Can you work these out from the model? Positions are in its coordinate system, mm. A direction names the side the tool comes from. Give positions to 0.01 mm unless a question says otherwise; leave off trailing zeros. Order: outer loops, then holes, each group sorted by start corner. A loop starts at its lowest first (then second) coordinate and runs counter-clockwise, first axis right, second up. Notation, with made-up numbers: (-18.75, 33.5) - (-5.75, 33.5) arc R16 ccw to (-5.75, 56.5) - close; hole circle Ø7 at (-10, 3.25). An arc over 180 degrees is marked (long way). One line per question, with ' | ' between items.
```python
from build123d import *

# Parameters (mm, degrees)
PAD012_DEPTH            = 3
FILLET037_R             = 3.35
SKETCH185_R             = 1.15
POCKET053_DEPTH         = 3
POCKET056_DEPTH         = 5
SKETCH189_W             = 32
SKETCH189_H             = 20
POCKET057_DEPTH         = 1.5
BODY024_PLACEMENT_ANGLE = 149


with BuildPart() as part:
    # Sketch184 → Pad012 (new body)
    with BuildSketch(Plane(origin=(0, 0, 0), x_dir=(1, 0, 0), z_dir=(0, 0, -1))):
        Polygon((101.467362, -402.500006), (130.400002, -402.500006), (135.400002, -402.500006), (135.400002, -397.500006), (174.999975, -357.90402), (174.999975, -245), (289.999995, -245), (294.999995, -245), (294.999995, -215), (289.999995, -215), (224.999995, -215), (224.999995, -199.999997), (219.999995, -199.999997), (199.999995, -199.999997), (194.999995, -199.999997), (194.999995, -215.000003), (168.459985, -215.000003), (161.999993, -198.359996), (161.999993, -115.000006), (161.999993, -110.000006), (156.999993, -110.000006), (134.576923, -122.534363), (131.999997, -126.895911), (131.999997, -200.027011), (144.989344, -239.967928), (144.989344, -343.839368), (96.467362, -392.500006), (96.467362, -397.500006), (96.467362, -402.500006), align=None)
    extrude(amount=PAD012_DEPTH)

    # Fillet037
    fillet037_edges = [part.edges().sort_by_distance(p)[0] for p in [
        (194.999995, 215.000003, -1.5),
        (168.459985, 215.000003, -1.5),
        (161.999993, 198.359996, -1.5),
        (161.999993, 110.000006, -1.5),
        (156.999993, 110.000006, -1.5),
        (134.576923, 122.534363, -1.5),
        (131.999997, 126.895911, -1.5),
        (131.999997, 200.027011, -1.5),
        (144.989344, 239.967928, -1.5),
        (144.989344, 343.839368, -1.5),
        (96.467362, 392.500006, -1.5),
        (135.400002, 397.500006, -1.5),
        (174.999975, 357.90402, -1.5),
        (174.999975, 245, -1.5),
        (294.999995, 245, -1.5),
        (294.999995, 215, -1.5),
        (224.999995, 215, -1.5),
    ]]
    fillet(fillet037_edges, radius=FILLET037_R)

    # Sketch185 (on Face5 of Fillet037) → Pocket053 (cut)
    with BuildSketch(Plane(origin=(0, 0, -3), x_dir=(1, 0, 0), z_dir=(0, 0, -1))):
        with Locations((105, -389)):
            Circle(SKETCH185_R)
        with Locations((145, -349)):
            Circle(SKETCH185_R)
        with Locations((147.500002, -309.000005)):
            Circle(SKETCH185_R)
        with Locations((147.500002, -259.000004)):
            Circle(SKETCH185_R)
        with Locations((172.500003, -259.000004)):
            Circle(SKETCH185_R)
        with Locations((172.500003, -309.000005)):
            Circle(SKETCH185_R)
        with Locations((172.500003, -349.000005)):
            Circle(SKETCH185_R)
        with Locations((147.665007, -382.765018)):
            Circle(SKETCH185_R)
        with Locations((178.000003, -242.500004)):
            Circle(SKETCH185_R)
        with Locations((218.000003, -242.500004)):
            Circle(SKETCH185_R)
        with Locations((258.000004, -242.500004)):
            Circle(SKETCH185_R)
        with Locations((258.000004, -217.500003)):
            Circle(SKETCH185_R)
        with Locations((292, -242.500004)):
            Circle(SKETCH185_R)
        with Locations((292.000004, -217.500003)):
            Circle(SKETCH185_R)
        with Locations((292.500004, -230.000003)):
            Circle(SKETCH185_R)
        with Locations((223.000003, -217.000003)):
            Circle(SKETCH185_R)
        with Locations((197, -217)):
            Circle(SKETCH185_R)
        with Locations((166.109996, -217.109995)):
            Circle(SKETCH185_R)
        with Locations((147.500002, -239)):
            Circle(SKETCH185_R)
        with Locations((141, -220)):
            Circle(SKETCH185_R)
        with Locations((134.427551, -201)):
            Circle(SKETCH185_R)
        with Locations((160.149996, -200.999996)):
            Circle(SKETCH185_R)
        with Locations((134.427551, -161)):
            Circle(SKETCH185_R)
        with Locations((159.500002, -161.000002)):
            Circle(SKETCH185_R)
        with Locations((137, -124)):
            Circle(SKETCH185_R)
        with Locations((146.849997, -118.149997)):
            Circle(SKETCH185_R)
        with Locations((159, -113)):
            Circle(SKETCH185_R)
    extrude(amount=-POCKET053_DEPTH, mode=Mode.SUBTRACT)

    # Sketch188 (on Face5 of Pocket053) → Pocket056 (cut)
    with BuildSketch(Plane(origin=(0, 0, -3), x_dir=(1, 0, 0), z_dir=(0, 0, -1))):
        Polygon((145, -269), (175, -269), (176, -269), (176, -410), (90, -410), (90, -269), align=None)
    extrude(amount=-POCKET056_DEPTH, mode=Mode.SUBTRACT)

    # Sketch189 (on Face2 of Pocket056) → Pocket057 (cut)
    with BuildSketch(Plane.XY):
        with Locations((160, 259)):
            Rectangle(SKETCH189_W, SKETCH189_H)
    extrude(amount=-POCKET057_DEPTH, mode=Mode.SUBTRACT)


with BuildPart() as part_1:
    # Body024 placement: moved
    add(part.part.moved(Location((707.641298, 2.853319, 22))).rotate(Axis((707.641298, 2.853319, 22), (0, 0, 1)), BODY024_PLACEMENT_ANGLE))


solid = part_1.part
```
(1) On a 3-axis mill with a long thin cutter (end or side, diameter ignored), from which of +Z, -Z, +X, -X, +Y, -Y can I reach the whole of each face in a straight line? I mean faces 1 (the face through (488.366, -47.542, 20.521)), 2 (the face through (442.435, -128.286, 21.26)), 3 (the face through (434.53, -73.07, 20.52)), 4 (the face through (426, -89, 19)). Say none if no direction works.
Answer below:
face 1: +Z, -Z, +Y | face 2: +Z, -X, -Y | face 3: +Z, -Z | face 4: -Z, +X, -X, +Y, -Y
(2) Imagine slicing it at D-D (y = -108.5). List the corners of the cut face in (x, z) for me.
Answer below:
outline: (417.27, 19) - (482.4, 19) - (482.4, 22) - (417.27, 22) - close
(3) Imagine slicing it at C-C (x = 387). List the corners of the cut face in (y, z) for me.
Answer below:
outline: (-90.31, 19) - (-55.31, 19) - (-55.31, 22) - (-90.31, 22) - close
(4) Imagine slicing it at B-B (z = 19.5). Count the separate pieces of the cut face and the enclosed holes in it, and give its area (3 significant figures).
Answer below:
separate pieces: 1 | enclosed holes: 21 | area: 8,670 mm^2
(5) Imagine slicing it at A-A (y = -60.5). List the corners of the cut face in (x, z) for me.
Answer below:
outline: (337.39, 19) - (395.63, 19) - (395.63, 22) - (337.39, 22) - close; (407.08, 19) - (424.76, 19) - (424.76, 22) - (407.08, 22) - close; (480.58, 19) - (515.58, 19) - (515.58, 22) - (480.58, 22) - close
(6) Will these pins go through, and if not, where does the flat tip stop? pin 1 (1.4 mm diameter, centred on x = 453.44, y = -97.69, fed in from -Z); pin 2 (1.5 mm diameter, centred on y = -86, z = 20.5, fed in from -X); pin 3 (1.5 mm diameter, centred on y = -37, z = 19.5, fed in from -X).
Answer below:
pin 1: through | pin 2: x = 378.58 | pin 3: x = 339.09
(7) If I drill on line 1 (X direction, y = -33, z = 21.75); line 2 (Y direction, x = 426.5, z = 20.05); line 3 (X direction, y = -61, z = 20.55), over which ranges is the centre line in solid material (lowest first)?
Answer below:
line 1: 341.94 to 344.19, 346.46 to 349.87, 497.1 to 525.2, 527.49 to 529.09 | line 2: -142.04 to -131.45, -129.16 to -125.26, -114.05 to -82.72, -80.66 to -61.55 | line 3: 338.22 to 396.47, 406.78 to 425.59, 480.28 to 515.28
(8) If we mould it in two halves opening along X, with no side actions, what happens to faces 5 (the face through (453.89, -137.95, 20.19)), 6 (the face through (373.665, -47.3, 20.521)), 7 (the face through (460.14, -88.76, 20.52)), 8 (the face through (424.335, -128.867, 19.854))? For each: released by +X, released by -X, zero draft, split by the parting line, or undercut.
Answer below:
face 5: released by +X | face 6: undercut | face 7: undercut | face 8: released by -X
